Part model, mm, in its own coordinate system. Face numbers are marked on the shaded views. A direction names the side the tool comes from. Round coordinates to 2 decimals unless told otherwise and drop trailing zeros. Write each loop counter-clockwise with the first axis right and the second up, starting at its lowest first coordinate (ties: lowest second). Pieces come first, ordered by that corner, then holes. Notation, with made-up numbers: (-17, 41) -> (21, 41) arc R18 cw to (21, 66) -> close; hole circle Ø3 at (76, 0). An arc over 180 degrees is marked (long way). Return JSON: item names as keys, results as strings. Group by question number.
(1) Tool access for the marked faces 1 and 2: list every direction of +Z, -Z, +X, -X, +Y, -Y with a clear straight run to the whole face (end or side of a thin tool).
(2) Saw through at C-C (z = 0). List the corners of the cut face in (x, y).
(3) Mould opens along X. For the marked faces 3, 4, 5 and 6 say: +X half, -X half, draft (parallel to the pull), parting line (faces both ways), or undercut.
(4) Saw through at B-B (x = 0). List the corners of the cut face in (y, z), plus the area to 3 significant figures.
(5) Saw through at A-A (y = 32). List the corners of the cut face in (x, z).
(6) Drop a flat-ended pin along its axis: pin 1 Ø10 at (x, z) = (16, 21.5) entering from +Y. Give the stop position or say it passes through.
(7) Drill centre lines: L1, parallel to X at y = 25, z = 30; L2, parallel to Y at x = 14.5, z = -11. Where is each one in solid material? Low to high. Write a range as from..to.
(8) Saw through at D-D (x = 28.5). List the corners of the cut face in (y, z), plus the area to 3 significant figures.
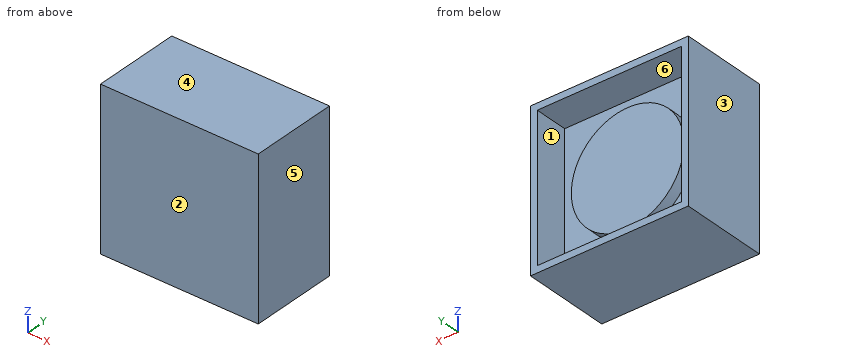
from build123d import *

# Parameters (mm, degrees)
SKETCH1_W           = 70
SKETCH1_H           = 70
BOSS_EXTRUDE1_DEPTH = 39
SKETCH2_W           = 64
SKETCH2_H           = 64
CUT_EXTRUDE1_DEPTH  = 15
SKETCH3_R           = 25
BOSS_EXTRUDE2_DEPTH = 5


with BuildPart() as part:
    # Sketch1 → Boss-Extrude1 (new body)
    with BuildSketch(Plane(origin=(0, 0, 0), x_dir=(1, 0, 0), z_dir=(0, 1, 0))):
        Rectangle(SKETCH1_W, SKETCH1_H)
    extrude(amount=BOSS_EXTRUDE1_DEPTH)

    # Sketch2 → Cut-Extrude1 (cut)
    with BuildSketch(Plane(origin=(0, 39, 0), x_dir=(1, 0, 0), z_dir=(0, 1, 0))):
        Rectangle(SKETCH2_W, SKETCH2_H)
    extrude(amount=-CUT_EXTRUDE1_DEPTH, mode=Mode.SUBTRACT)

    # Sketch3 → Boss-Extrude2 (add)
    with BuildSketch(Plane(origin=(0, 24, 0), x_dir=(1, 0, 0), z_dir=(0, 1, 0))):
        with Locations(Location((0, 0, 0), (0, 0, 90))):
            Circle(SKETCH3_R)
    extrude(amount=BOSS_EXTRUDE2_DEPTH)


solid = part.part
Computed values:
{
 "1": {"face 1": "+Y", "face 2": "+Z, -Z, +X, -X, -Y"},
 "2": {"outline": "(-35, 0) -> (35, 0) -> (35, 39) -> (32, 39) -> (32, 24) -> (25, 24) -> (25, 29) -> (-25, 29) -> (-25, 24) -> (-32, 24) -> (-32, 39) -> (-35, 39) -> close"},
 "3": {"face 3": "-X half", "face 4": "draft", "face 5": "+X half", "face 6": "undercut"},
 "4": {"outline": "(0, -35) -> (39, -35) -> (39, -32) -> (24, -32) -> (24, -25) -> (29, -25) -> (29, 25) -> (24, 25) -> (24, 32) -> (39, 32) -> (39, 35) -> (0, 35) -> close", "area": "2,020 mm2"},
 "5": {"outline": "(-35, -35) -> (35, -35) -> (35, 35) -> (-35, 35) -> close; hole (-32, -32) -> (32, -32) -> (32, 32) -> (-32, 32) -> close"},
 "6": {"pin 1": "y = 29"},
 "7": {"L1": "-35..-32, 32..35", "L2": "0..29"},
 "8": {"outline": "(0, -35) -> (39, -35) -> (39, -32) -> (24, -32) -> (24, 32) -> (39, 32) -> (39, 35) -> (0, 35) -> close", "area": "1,770 mm2"}
}
